Verification items for the finished model (mm, model axes). Face numbers are marked on the shaded views. A direction names the side the tool comes from. Coordinates: 2 decimals unless noted, no trailing zeros. Write each loop counter-clockwise with the first axis right and the second up, starting at its lowest first coordinate (ties: lowest second). Pieces come first, ordered by that corner, then holes. Notation, with made-up numbers: M -9.75,22 L 33.25,22 A22 ccw 33.25,29 Z; hole C 30,-25.75 d10. An arc over 180 degrees is marked long. One line per item, written item: value.
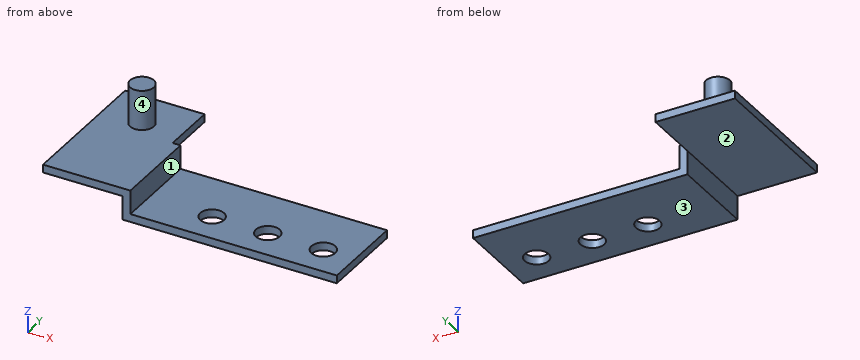
```python
from build123d import *

# Parameters (mm, degrees)
PAD_DEPTH       = 18
SKETCH001_W     = 27
SKETCH001_H     = 7
POCKET_DEPTH    = 10
SKETCH002_W     = 1
SKETCH002_H     = 7
POCKET001_DEPTH = 4.001
SKETCH003_R     = 1.5
POCKET002_DEPTH = 1.001
SKETCH004_R     = 1.5
PAD001_DEPTH    = 6


with BuildPart() as body:
    # Sketch → Pad (new body)
    with BuildSketch(Plane.XZ):
        Polygon((0, 0), (27, 0), (27, 1), (1, 1), (1, 4), (-10, 4), (-10, 3), (0, 3), align=None)
    extrude(amount=PAD_DEPTH)

    # Sketch001 (on Face3 of Pad) → Pocket (cut)
    with BuildSketch(Plane(origin=(0, 0, 1), x_dir=(-1, 0, 0), z_dir=(0, 0, 1))):
        with Locations((-13.5, 14.5)):
            Rectangle(SKETCH001_W, SKETCH001_H)
    extrude(amount=-POCKET_DEPTH, mode=Mode.SUBTRACT)

    # Sketch002 (on Face8 of Pocket) → Pocket001 (cut, through all)
    with BuildSketch(Plane(origin=(0, 0, 4), x_dir=(-1, 0, 0), z_dir=(0, 0, 1))):
        with Locations((-0.5, 14.5)):
            Rectangle(SKETCH002_W, SKETCH002_H)
    extrude(amount=-POCKET001_DEPTH, mode=Mode.SUBTRACT)

    # Sketch003 (on Face7 of Pocket001) → Pocket002 (cut, through all)
    with BuildSketch(Plane(origin=(0, 0, 1), x_dir=(-1, 0, 0), z_dir=(0, 0, 1))):
        with Locations((-23, 4)):
            Circle(SKETCH003_R)
        with Locations((-16, 4)):
            Circle(SKETCH003_R)
        with Locations((-9, 4)):
            Circle(SKETCH003_R)
    extrude(amount=-POCKET002_DEPTH, mode=Mode.SUBTRACT)

    # Sketch004 (on Face14 of Pocket002) → Pad001 (join)
    with BuildSketch(Plane(origin=(0, 0, 3), x_dir=(1, 0, 0), z_dir=(0, 0, -1))):
        with Locations((-5, 13)):
            Circle(SKETCH004_R)
    extrude(amount=-PAD001_DEPTH)


with BuildPart() as part_mirroring:
    # Part__Mirroring: instance of Body
    add(body.part.mirror(Plane(origin=(0, 0, 0), x_dir=(1, 0, 0), z_dir=(0, 1, 0))))


solid = part_mirroring.part
```
Item 1: Cross-section at D-D, the plane x = -5. Enter the section's corners in (y, z).
The answers:
outline: M 0,3 L 18,3 L 18,4 L 14.5,4 L 14.5,9 L 11.5,9 L 11.5,4 L 0,4 Z
Item 2: Cross-section at A-A, the plane y = 4. Enter the section's corners in (x, z).
The answers:
outline: M -10,3 L 0,3 L 0,0 L 7.5,0 L 7.5,1 L 1,1 L 1,4 L -10,4 Z; M 10.5,0 L 14.5,0 L 14.5,1 L 10.5,1 Z; M 17.5,0 L 21.5,0 L 21.5,1 L 17.5,1 Z; M 24.5,0 L 27,0 L 27,1 L 24.5,1 Z
Item 3: Scan lines: line 1 (Y direction, x = 16, z = 0.55); line 2 (X direction, y = 10.5, z = 0.5); line 3 (Z direction, x = -1, y = 4.5). Record each from-to range of solid material in increasing order.
The answers:
line 1: y = 0 to 2.5, 5.5 to 11
line 2: x = 0 to 27
line 3: z = 3 to 4
Item 4: Cross-section at B-B, the plane x = 9. Enter the section's corners in (y, z).
The answers:
outline: M 0,0 L 2.5,0 L 2.5,1 L 0,1 Z; M 5.5,0 L 11,0 L 11,1 L 5.5,1 Z
Item 5: Go/stop test with flat-tipped pins: P1, Ø5, axis at x = -5.5, y = 7.5, coming from the -Z side; P2, Ø9, axis at x = 13, y = 3.5, coming from the +Z side; P3, Ø0.5, axis at y = 15.5, z = 3.5, coming from the +X side. Record where each tip stops, or that it passes through.
The answers:
P1: stops at z = 3
P2: stops at z = 1
P3: stops at x = 0
Item 6: Cross-section at C-C, the plane y = 9.5. Enter the section's corners in (x, z), and give its area (3 significant figures).
The answers:
outline: M -10,3 L 0,3 L 0,0 L 27,0 L 27,1 L 1,1 L 1,4 L -10,4 Z
area: 40.0 mm²
Item 7: Access from +Z, -Z, +X, -X, +Y, -Y to the whole of each face (thin tool, end or side, straight path). Record for the marked faces 1, 2, 3 and 4.
The answers:
face 1: +Z, +X, +Y, -Y
face 2: -Z, -X, +Y, -Y
face 3: -Z, +X, -X, +Y, -Y
face 4: +Z
